Here's how the part is built. I have some questions about the finished solid (model axes, mm). A direction names the side the tool comes from. Round coordinates to 2 decimals unless told otherwise and drop trailing zeros. Order: outer loops, then holes, each group sorted by start corner. A loop starts at its lowest first (then second) coordinate and runs counter-clockwise, first axis right, second up. Notation, with made-up numbers: (54.5, 88.5) -> (77.5, 88.5) arc R27 cw to (77.5, 127.5) -> close; hole circle Ø5 at (34.5, 27.5). An arc over 180 degrees is marked (long way). One line per item, written item: value.
```python
from build123d import *

# Parameters (mm, degrees)
SKETCH1_R           = 3
BOSS_EXTRUDE1_DEPTH = 9.2
FILLET1_R           = 0.1
SKETCH4_R           = 3
BOSS_EXTRUDE4_DEPTH = 7.1
SKETCH6_R           = 1.75
BOSS_EXTRUDE6_DEPTH = 0.4
BOSS_EXTRUDE5_DEPTH = 3.1
SKETCH7_R           = 0.25
BOSS_EXTRUDE7_DEPTH = 3


with BuildPart() as part:
    # Sketch1 → Boss-Extrude1 (new body)
    with BuildSketch(Plane(origin=(0, 0, 0), x_dir=(1, 0, 0), z_dir=(0, 1, 0))):
        with Locations(Location((0, 0, 0), (0, 0, 270))):
            Circle(SKETCH1_R)
    extrude(amount=BOSS_EXTRUDE1_DEPTH)

    # Fillet1
    fillet1_edges = [part.edges().sort_by_distance(p)[0] for p in [
        (0, 9.2, -3),
    ]]
    fillet(fillet1_edges, radius=FILLET1_R)

    # Sketch4 → Boss-Extrude4 (add)
    with BuildSketch(Plane(origin=(0, 9.2, 0), x_dir=(1, 0, 0), z_dir=(0, 1, 0))):
        with Locations(Location((0, 0, 0), (0, 0, 270))):
            Circle(SKETCH4_R)
    extrude(amount=BOSS_EXTRUDE4_DEPTH)

    # Sketch6 → Boss-Extrude6 (add)
    with BuildSketch(Plane(origin=(0, 16.3, 0), x_dir=(1, 0, 0), z_dir=(0, 1, 0))):
        with Locations(Location((0, 0, 0), (0, 0, 270))):
            Circle(SKETCH6_R)
    extrude(amount=BOSS_EXTRUDE6_DEPTH)

    # Sketch5 → Boss-Extrude5 (add)
    with BuildSketch(Plane(origin=(0, 16.3, 0), x_dir=(1, 0, 0), z_dir=(0, 1, 0))):
        with BuildLine():
            Line((-0.866025404, -0.5), (0, -0.5))
            Line((0, -0.5), (0.866025404, -0.5))
            ThreePointArc((0.866025404, -0.5), (0, 1), (-0.866025404, -0.5))
        make_face()
    extrude(amount=BOSS_EXTRUDE5_DEPTH)

    # Sketch7 → Boss-Extrude7 (add)
    with BuildSketch(Plane.XZ):
        with Locations(Location((-1.6, 0, 0), (0, 0, 90))):
            Circle(SKETCH7_R)
        with Locations(Location((1.6, 0, 0), (0, 0, 90))):
            Circle(SKETCH7_R)
    extrude(amount=BOSS_EXTRUDE7_DEPTH)


solid = part.part
```
Q1. I want a section at C-C on y = 14.5. Write out the boundary of the cut face in (x, z).
Answers:
outline: circle Ø6 at (0, 0)
Q2. I want a section at B-B on x = 0. Write out the boundary of the cut face in (y, z).
Answers:
outline: (0, -3) -> (9.1, -3) arc R0.1 ccw to (9.2, -2.9) -> (9.2, -3) -> (16.3, -3) -> (16.3, -1.75) -> (16.7, -1.75) -> (16.7, -1) -> (19.4, -1) -> (19.4, 0.5) -> (16.7, 0.5) -> (16.7, 1.75) -> (16.3, 1.75) -> (16.3, 3) -> (9.2, 3) -> (9.2, 2.9) arc R0.1 ccw to (9.1, 3) -> (0, 3) -> close
Q3. I need wall thicknesses on line 1 along Y through (x, z) = (1.25, -2.25); line 2 along X through (y, z) = (17.5, 0); line 3 along X through (y, z) = (2.5, -0.75). Which ranges of each line are inside material? Lowest first, please.
Answers:
line 1: 0 to 16.3
line 2: -1 to 1
line 3: -2.9 to 2.9
Q4. For P1, Ø3, axis at x = -0.5, y = 0.5, coming from the -Z side; P2, Ø2, axis at x = 1, z = 2.5, coming from the -Y side; P3, Ø0.5, axis at x = 0.5, y = 18.5, coming from the +Z side; P4, Ø1.5, axis at x = -1.5, y = 0, coming from the -Z side, each with a flat end and sliding along its axis, tell me the tip position at first contact or that it passes through.
Answers:
P1: z = -3
P2: y = 0
P3: z = 0.5
P4: z = -2.9
Q5. I want a section at A-A on z = 0. Write out the boundary of the cut face in (x, y), then the cut area to 3 significant figures.
Answers:
outline: (-3, 0) -> (-1.85, 0) -> (-1.85, -3) -> (-1.35, -3) -> (-1.35, 0) -> (1.35, 0) -> (1.35, -3) -> (1.85, -3) -> (1.85, 0) -> (3, 0) -> (3, 9.1) arc R0.1 ccw to (2.9, 9.2) -> (3, 9.2) -> (3, 16.3) -> (1.75, 16.3) -> (1.75, 16.7) -> (1, 16.7) -> (1, 19.4) -> (-1, 19.4) -> (-1, 16.7) -> (-1.75, 16.7) -> (-1.75, 16.3) -> (-3, 16.3) -> (-3, 9.2) -> (-2.9, 9.2) arc R0.1 ccw to (-3, 9.1) -> close
area: 108 mm2
Q6. Which directions (+Z, -Z, +X, -X, +Y, -Y) give clear straight access to the entire face, cutting with the end or side of a thin tool? Please do faces 1 (the face through (0.9, 4.49, 2.86)), 2 (the face through (0, 18, 0.5)), 3 (the face through (-1.71, 16.5, -0.38)).
Answers:
face 1: +Y, -Y
face 2: +Z, +X, -X, +Y
face 3: +Y
